```python
from build123d import *

# Parameters (mm, degrees)
SKETCH1_W           = 210.6422
SKETCH1_H           = 109.1692
BOSS_EXTRUDE1_DEPTH = 5.7658
SKETCH2_W           = 210.6422
SKETCH2_H           = 109.1692
SKETCH2_W_2         = 13.081
SKETCH2_H_2         = 13.081
SKETCH2_W_3         = 156.083
SKETCH2_H_3         = 88.0872
BOSS_EXTRUDE2_DEPTH = 1.27
CUT_EXTRUDE1_REACH  = 120.834
SKETCH3_R           = 1.3462
SKETCH3_3_R         = 1.3462
BOSS_EXTRUDE3_DEPTH = 7.0358
FILLET1_R           = 2.54
CUT_EXTRUDE2_REACH  = 122.497
SKETCH4_R           = 1.3462
SKETCH4_3_R         = 1.3462
BOSS_EXTRUDE4_DEPTH = 7.0358


with BuildPart() as part:
    # Sketch1 → Boss-Extrude1 (new body)
    with BuildSketch(Plane.XY):
        Rectangle(SKETCH1_W, SKETCH1_H)
        with BuildLine():
            Line((45.6565, 49.7078), (45.6565, 51.4096))
            Line((45.6565, 51.4096), (-42.2275, 51.4096))
            Line((-42.2275, 51.4096), (-42.2275, 49.7078))
            ThreePointArc((-42.2275, 49.7078), (-45.4025, 46.5328), (-48.5775, 49.7078))
            Line((-48.5775, 49.7078), (-48.5775, 51.4096))
            Line((-48.5775, 51.4096), (-73.9775, 51.4096))
            Line((-73.9775, 51.4096), (-73.9775, 49.7078))
            ThreePointArc((-73.9775, 49.7078), (-77.1525, 46.5328), (-80.3275, 49.7078))
            Line((-80.3275, 49.7078), (-80.3275, 51.4096))
            Line((-80.3275, 51.4096), (-102.1461, 51.4096))
            Line((-102.1461, 51.4096), (-102.1461, 17.1069))
            Line((-102.1461, 17.1069), (-84.9757, 17.1069))
            ThreePointArc((-84.9757, 17.1069), (-80.7085, 12.8397), (-84.9757, 8.5725))
            Line((-84.9757, 8.5725), (-102.1461, 8.5725))
            Line((-102.1461, 8.5725), (-102.1461, -8.5725))
            Line((-102.1461, -8.5725), (-84.9757, -8.5725))
            ThreePointArc((-84.9757, -8.5725), (-80.7085, -12.8397), (-84.9757, -17.1069))
            Line((-84.9757, -17.1069), (-102.1461, -17.1069))
            Line((-102.1461, -17.1069), (-102.1461, -51.4096))
            Line((-102.1461, -51.4096), (-78.509915544, -51.4096))
            ThreePointArc((-78.509915544, -51.4096), (-77.1525, -51.1048), (-75.795084456, -51.4096))
            Line((-75.795084456, -51.4096), (-46.759915544, -51.4096))
            ThreePointArc((-46.759915544, -51.4096), (-45.4025, -51.1048), (-44.045084456, -51.4096))
            Line((-44.045084456, -51.4096), (47.474084456, -51.4096))
            ThreePointArc((47.474084456, -51.4096), (48.8315, -51.1048), (50.188915544, -51.4096))
            Line((50.188915544, -51.4096), (79.224084456, -51.4096))
            ThreePointArc((79.224084456, -51.4096), (80.5815, -51.1048), (81.938915544, -51.4096))
            Line((81.938915544, -51.4096), (102.1461, -51.4096))
            Line((102.1461, -51.4096), (102.1461, -17.1069))
            Line((102.1461, -17.1069), (88.4047, -17.1069))
            ThreePointArc((88.4047, -17.1069), (84.1375, -12.8397), (88.4047, -8.5725))
            Line((88.4047, -8.5725), (102.1461, -8.5725))
            Line((102.1461, -8.5725), (102.1461, 8.5725))
            Line((102.1461, 8.5725), (88.4047, 8.5725))
            ThreePointArc((88.4047, 8.5725), (84.1375, 12.8397), (88.4047, 17.1069))
            Line((88.4047, 17.1069), (102.1461, 17.1069))
            Line((102.1461, 17.1069), (102.1461, 51.4096))
            Line((102.1461, 51.4096), (83.7565, 51.4096))
            Line((83.7565, 51.4096), (83.7565, 49.7078))
            ThreePointArc((83.7565, 49.7078), (80.5815, 46.5328), (77.4065, 49.7078))
            Line((77.4065, 49.7078), (77.4065, 51.4096))
            Line((77.4065, 51.4096), (52.0065, 51.4096))
            Line((52.0065, 51.4096), (52.0065, 49.7078))
            ThreePointArc((52.0065, 49.7078), (48.8315, 46.5328), (45.6565, 49.7078))
        make_face(mode=Mode.SUBTRACT)
    extrude(amount=BOSS_EXTRUDE1_DEPTH)

    # Sketch2 → Boss-Extrude2 (add)
    with BuildSketch(Plane.XY.offset(5.7658)):
        Rectangle(SKETCH2_W, SKETCH2_H)
        with Locations((92.8243, 25.6794)):
            Rectangle(SKETCH2_W_2, SKETCH2_H_2, mode=Mode.SUBTRACT)
        with Locations((92.8243, 0)):
            Rectangle(SKETCH2_W_2, SKETCH2_H_2, mode=Mode.SUBTRACT)
        with Locations((92.8243, -25.6794)):
            Rectangle(SKETCH2_W_2, SKETCH2_H_2, mode=Mode.SUBTRACT)
        with Locations((-92.8243, -25.6794)):
            Rectangle(SKETCH2_W_2, SKETCH2_H_2, mode=Mode.SUBTRACT)
        Rectangle(SKETCH2_W_3, SKETCH2_H_3, mode=Mode.SUBTRACT)
        with Locations((-92.8243, 0)):
            Rectangle(SKETCH2_W_2, SKETCH2_H_2, mode=Mode.SUBTRACT)
        with Locations((-92.8243, 25.6794)):
            Rectangle(SKETCH2_W_2, SKETCH2_H_2, mode=Mode.SUBTRACT)
    extrude(amount=BOSS_EXTRUDE2_DEPTH)

    # Sketch3 → Cut-Extrude1 (cut, up to next)
    with BuildSketch(Plane.XY, mode=Mode.PRIVATE) as cut_extrude1_sk1:
        with Locations((0, 54.5846)):
            Circle(SKETCH3_R)
    cut_extrude1_tool1 = extrude(cut_extrude1_sk1.sketch, amount=CUT_EXTRUDE1_REACH, mode=Mode.PRIVATE) & part.part
    # Sketch3 → Cut-Extrude1 (cut, up to next)
    with BuildSketch(Plane.XY, mode=Mode.PRIVATE) as cut_extrude1_sk2:
        with Locations((76.2, 54.5846)):
            Circle(SKETCH3_R)
    cut_extrude1_tool2 = extrude(cut_extrude1_sk2.sketch, amount=CUT_EXTRUDE1_REACH, mode=Mode.PRIVATE) & part.part
    # Sketch3 → Cut-Extrude1 (cut, up to next)
    with BuildSketch(Plane.XY, mode=Mode.PRIVATE) as cut_extrude1_sk3:
        with Locations((-76.2, 54.5846)):
            Circle(SKETCH3_R)
    cut_extrude1_tool3 = extrude(cut_extrude1_sk3.sketch, amount=CUT_EXTRUDE1_REACH, mode=Mode.PRIVATE) & part.part
    cut_extrude1_1 = cut_extrude1_tool1.solids().sort_by_distance((0, 54.5846, 0))[0]
    add(cut_extrude1_1, mode=Mode.SUBTRACT)
    cut_extrude1_2 = cut_extrude1_tool2.solids().sort_by_distance((76.2, 54.5846, 0))[0]
    add(cut_extrude1_2, mode=Mode.SUBTRACT)
    cut_extrude1_3 = cut_extrude1_tool3.solids().sort_by_distance((-76.2, 54.5846, 0))[0]
    add(cut_extrude1_3, mode=Mode.SUBTRACT)
    cut_extrude1 = cut_extrude1_1 + cut_extrude1_2 + cut_extrude1_3  # Cut-Extrude1 as one shape, for the pattern or mirror that repeats it

    # Sketch3<3> → Boss-Extrude3 (add)
    # profile 1 of 3: a face of its own
    with BuildSketch(Plane.XY):
        with BuildLine():
            Line((5.001994598, 54.5846), (5.001994598, 52.2986))
            Line((5.001994598, 52.2986), (-5.001994598, 52.2986))
            Line((-5.001994598, 52.2986), (-5.001994598, 54.5846))
            ThreePointArc((-5.001994598, 54.5846), (-3.97669446, 54.910001078), (-3.326685403, 55.767097608))
            ThreePointArc((-3.326685403, 55.767097608), (0, 58.1152), (3.326685403, 55.767097608))
            ThreePointArc((3.326685403, 55.767097608), (3.97669446, 54.910001078), (5.001994598, 54.5846))
        make_face()
        with Locations(Location((0, 54.5846, 0), (0, 0, 180))):
            Circle(SKETCH3_3_R, mode=Mode.SUBTRACT)
    # profile 2 of 3: a face of its own
    with BuildSketch(Plane.XY):
        with BuildLine():
            Line((-81.201994598, 54.5846), (-81.201994598, 52.2986))
            Line((-81.201994598, 52.2986), (-71.198005402, 52.2986))
            Line((-71.198005402, 52.2986), (-71.198005402, 54.5846))
            ThreePointArc((-71.198005402, 54.5846), (-72.22330554, 54.910001078), (-72.873314597, 55.767097608))
            ThreePointArc((-72.873314597, 55.767097608), (-76.2, 58.1152), (-79.526685403, 55.767097608))
            ThreePointArc((-79.526685403, 55.767097608), (-80.17669446, 54.910001078), (-81.201994598, 54.5846))
        make_face()
        with Locations(Location((-76.2, 54.5846, 0), (0, 0, 180))):
            Circle(SKETCH3_3_R, mode=Mode.SUBTRACT)
    # profile 3 of 3: a face of its own
    with BuildSketch(Plane.XY):
        with BuildLine():
            Line((71.198005402, 54.5846), (71.198005402, 52.2986))
            Line((71.198005402, 52.2986), (81.201994598, 52.2986))
            Line((81.201994598, 52.2986), (81.201994598, 54.5846))
            ThreePointArc((81.201994598, 54.5846), (80.17669446, 54.910001078), (79.526685403, 55.767097608))
            ThreePointArc((79.526685403, 55.767097608), (76.2, 58.1152), (72.873314597, 55.767097608))
            ThreePointArc((72.873314597, 55.767097608), (72.22330554, 54.910001078), (71.198005402, 54.5846))
        make_face()
        with Locations(Location((76.2, 54.5846, 0), (0, 0, 180))):
            Circle(SKETCH3_3_R, mode=Mode.SUBTRACT)
    boss_extrude3 = extrude(amount=BOSS_EXTRUDE3_DEPTH)

    # Mirror1: Cut-Extrude1, Boss-Extrude3 across plane
    add(cut_extrude1.mirror(Plane.ZX), mode=Mode.SUBTRACT)
    add(boss_extrude3.mirror(Plane.ZX))

    # Fillet1
    fillet1_edges = [part.edges().sort_by_distance(p)[0] for p in [
        (-105.3211, 54.5846, 3.5179),
        (105.3211, 54.5846, 3.5179),
        (105.3211, -54.5846, 3.5179),
        (-105.3211, -54.5846, 3.5179),
    ]]
    fillet(fillet1_edges, radius=FILLET1_R)

    # Sketch4 → Cut-Extrude2 (cut, up to next)
    with BuildSketch(Plane.XY, mode=Mode.PRIVATE) as cut_extrude2_sk1:
        with Locations((105.3211, 0)):
            Circle(SKETCH4_R)
    cut_extrude2_tool1 = extrude(cut_extrude2_sk1.sketch, amount=CUT_EXTRUDE2_REACH, mode=Mode.PRIVATE) & part.part
    cut_extrude2 = cut_extrude2_tool1.solids().sort_by_distance((105.3211, 0, 0))[0]
    add(cut_extrude2, mode=Mode.SUBTRACT)

    # Sketch4<3> → Boss-Extrude4 (add)
    with BuildSketch(Plane.XY):
        with BuildLine():
            Line((105.3211, -5.001994598), (103.0351, -5.001994598))
            Line((103.0351, -5.001994598), (103.0351, 5.001994598))
            Line((103.0351, 5.001994598), (105.3211, 5.001994598))
            ThreePointArc((105.3211, 5.001994598), (105.646501078, 3.97669446), (106.503597608, 3.326685403))
            ThreePointArc((106.503597608, 3.326685403), (108.8517, 0), (106.503597608, -3.326685403))
            ThreePointArc((106.503597608, -3.326685403), (105.646501078, -3.97669446), (105.3211, -5.001994598))
        make_face()
        with Locations(Location((105.3211, 0, 0), (0, 0, 180))):
            Circle(SKETCH4_3_R, mode=Mode.SUBTRACT)
    boss_extrude4 = extrude(amount=BOSS_EXTRUDE4_DEPTH)

    # Mirror2: Cut-Extrude2, Boss-Extrude4 across plane
    add(cut_extrude2.mirror(Plane(origin=(0, 0, 0), x_dir=(0, 0, 1), z_dir=(1, 0, 0))), mode=Mode.SUBTRACT)
    add(boss_extrude4.mirror(Plane(origin=(0, 0, 0), x_dir=(0, 0, 1), z_dir=(1, 0, 0))))


solid = part.part
```
The listing builds one solid part. Answer for the finished solid, in the listing's coordinates (mm). A direction names the side the tool comes from. Give positions to 0.01 mm unless a question says otherwise; leave off trailing zeros. Order: outer loops, then holes, each group sorted by start corner. A loop starts at its lowest first (then second) coordinate and runs counter-clockwise, first axis right, second up. Notation, with made-up numbers: (0.5, -16.5) - (19.5, -16.5) arc R10 ccw to (19.5, -11.5) - close; hole circle Ø3 at (65.5, 23). An arc over 180 degrees is marked (long way). Answer in a Markdown table with one row per item. Add a question column.
Q1. Given P1, Ø4, axis at y = 16, z = 1.5, coming from the +X side; P2, Ø1, axis at x = 92, z = 6, coming from the -Y side; P3, Ø1.4, axis at y = 26, z = 6.5, coming from the -X side, each flat-ended and moving along its own axis, determine where each tip first touches the part or whether it passes through.
Q2. For a pull along X with two mould halves and no side action, classify faces 6 (the flat face through (92, -51.41, 3)), 7 (the cylindrical face through (-108.85, 0.06, 3.47)), 8 (the flat face through (-92, -54.585, 3)) as released by +X, released by -X, zero draft, split by the parting line, or undercut.
Q3. Find the intervals of material crossed by line 1 along X through (y, z) = (50.5, 5.5); line 2 along Y through (x, z) = (96.5, 0.5); line 3 along X through (y, z) = (-28.5, 6), in increasing order. Write a range as [from, to].
Q4. The part is cut by section C-C (y = -36). Determine the outline of the cut face in (x, z).
Q5. The part is cut by section A-A (x = -63.5). Determine the outline of the cut face in (y, z), then the cut area to 3 significant figures.
Q6. Which of the six approach directions +Z, -Z, +X, -X, +Y, -Y give full straight-line access (tool end or side, diameter ignored) to faces 1 (the flat face through (92, -54.585, 3)), 2 (the flat face through (102.146, -34, 3)), 3 (the flat face through (32, 52, 0)), 4 (the flat face through (-105.321, 28, 3)), 5 (the flat face through (92, 54.585, 3))?
Q7. The part is cut by section B-B (y = 21.5). Determine the outline of the cut face in (x, z).
Q8. The part is cut by section D-D (z = 2). Give the number of separate pieces and of enclosed holes in the cut face, then the cut area to 3 significant figures.
Determined:
| question | item | result |
|---|---|---|
| 1 | P1 | stops at x = 105.32 |
| 1 | P2 | stops at y = -54.58 |
| 1 | P3 | stops at x = -105.32 |
| 2 | face 6 | undercut |
| 2 | face 7 | released by -X |
| 2 | face 8 | zero draft |
| 3 | line 1 | x = [-105.32, -102.15], [-80.33, -73.98], [-48.58, -42.23], [45.66, 52.01], [77.41, 83.76], [102.15, 105.32] |
| 3 | line 2 | y = [-54.58, -51.41], [-17.11, -8.57], [8.57, 17.11], [51.41, 54.58] |
| 3 | line 3 | x = [-105.32, -99.36], [-86.28, -78.04], [78.04, 86.28], [99.36, 105.32] |
| 4 | outline | (-105.32, 0) - (-102.15, 0) - (-102.15, 5.77) - (-78.04, 5.77) - (-78.04, 7.04) - (-105.32, 7.04) - close; (78.04, 5.77) - (102.15, 5.77) - (102.15, 0) - (105.32, 0) - (105.32, 7.04) - (78.04, 7.04) - close |
| 5 | outline | (-54.58, 0) - (-51.41, 0) - (-51.41, 5.77) - (-44.04, 5.77) - (-44.04, 7.04) - (-54.58, 7.04) - close; (44.04, 5.77) - (51.41, 5.77) - (51.41, 0) - (54.58, 0) - (54.58, 7.04) - (44.04, 7.04) - close |
| 5 | area | 63.4 mm² |
| 6 | face 1 | +Z, -Z, +X, -Y |
| 6 | face 2 | -Z |
| 6 | face 3 | -Z, +X, -X, +Y, -Y |
| 6 | face 4 | +Z, -Z, -X, +Y |
| 6 | face 5 | +Z, -Z, +X, +Y |
| 7 | outline | (-105.32, 0) - (-102.15, 0) - (-102.15, 5.77) - (-99.36, 5.77) - (-99.36, 7.04) - (-105.32, 7.04) - close; (-86.28, 5.77) - (-78.04, 5.77) - (-78.04, 7.04) - (-86.28, 7.04) - close; (78.04, 5.77) - (86.28, 5.77) - (86.28, 7.04) - (78.04, 7.04) - close; (99.36, 5.77) - (102.15, 5.77) - (102.15, 0) - (105.32, 0) - (105.32, 7.04) - (99.36, 7.04) - close |
| 8 | separate pieces | 1 |
| 8 | enclosed holes | 9 |
| 8 | area | 2,850 mm² |
